from build123d import *

# Parameters (mm, degrees)
F0_W     = 50
F0_H     = 23
F0_R     = 2.21862
F1_DEPTH = 3.5
F2_R     = 1.5


with BuildPart() as f1:
    # F0 (on Front) → F1 (new body)
    with BuildSketch(Plane.XZ):
        Rectangle(F0_W, F0_H)
        with Locations((-19.98966, 0)):
            Circle(F0_R, mode=Mode.SUBTRACT)
    extrude(amount=F1_DEPTH)

    # F2
    f2_edges = [f1.edges().sort_by_distance(p)[0] for p in [
        (0, -3.5, -11.5),
        (-25, -3.5, 0),
        (25, -3.5, 0),
        (0, -3.5, 11.5),
    ]]
    fillet(f2_edges, radius=F2_R)


solid = f1.part
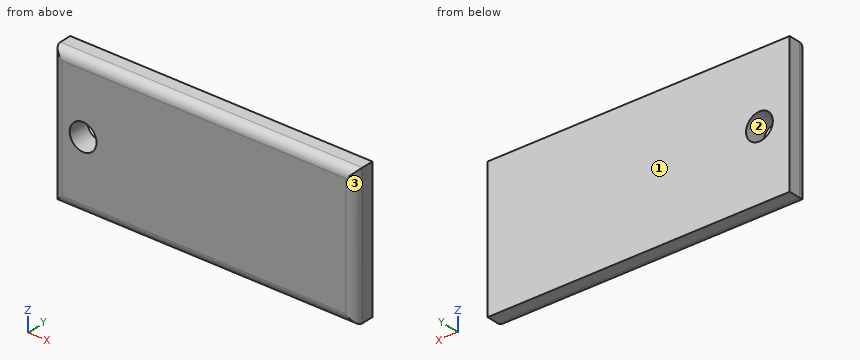
The listing builds one solid part. Answer for the finished solid, in the listing's coordinates (mm). Face numbers are marked on the shaded views. Give positions to 0.01 mm unless a question says otherwise; leave off trailing zeros. Loops run counter-clockwise (first coordinate to the right, second up) from the corner with the lowest first, then second, coordinate; pieces in that order, holes last.
Item 1: Each of these flat-tipped pins is pushed along its axis until it touches: pin 1 Ø4 at (x, z) = (-11.5, 4.5) entering from +Y; pin 2 Ø1 at (y, z) = (-3, 6.5) entering from +X. Where does it stop, or does it pass through?
Derived:
pin 1: stops at y = 0
pin 2: stops at x = 24.91
Item 2: Determine the mould class of the marked faces 1, 2 and 3 for opening direction X: +X half, -X half, draft (parallel to the pull), parting line (faces both ways), or undercut.
Derived:
face 1: draft
face 2: undercut
face 3: +X half
Item 3: A cutting plane is placed at B-B (y = -2.9). Give the vertices of the cut face in (x, z).
Derived:
outline: (-24.7, -11.2) - (24.7, -11.2) - (24.7, 11.2) - (-24.7, 11.2) - close; hole circle Ø4.44 at (-19.99, 0)
Item 4: A cutting plane is placed at A-A (z = 0). Give the vertices of the cut face in (x, y), then the cut area to 3 significant figures.
Derived:
outline: (-25, -2) arc R1.5 ccw to (-23.5, -3.5) - (-22.21, -3.5) - (-22.21, 0) - (-25, 0) - close; (-17.77, -3.5) - (23.5, -3.5) arc R1.5 ccw to (25, -2) - (25, 0) - (-17.77, 0) - close
area: 159 mm2
Item 5: Find the intervals of material crossed by line 1 along Z through (x, y) = (-19, -0.5); line 2 along X through (y, z) = (-1.3, -1.5); line 3 along Z through (x, y) = (7.5, -2.9), in increasing order.
Derived:
line 1: z = -11.5 to -1.99, 1.99 to 11.5
line 2: x = -25 to -21.62, -18.35 to 25
line 3: z = -11.2 to 11.2
